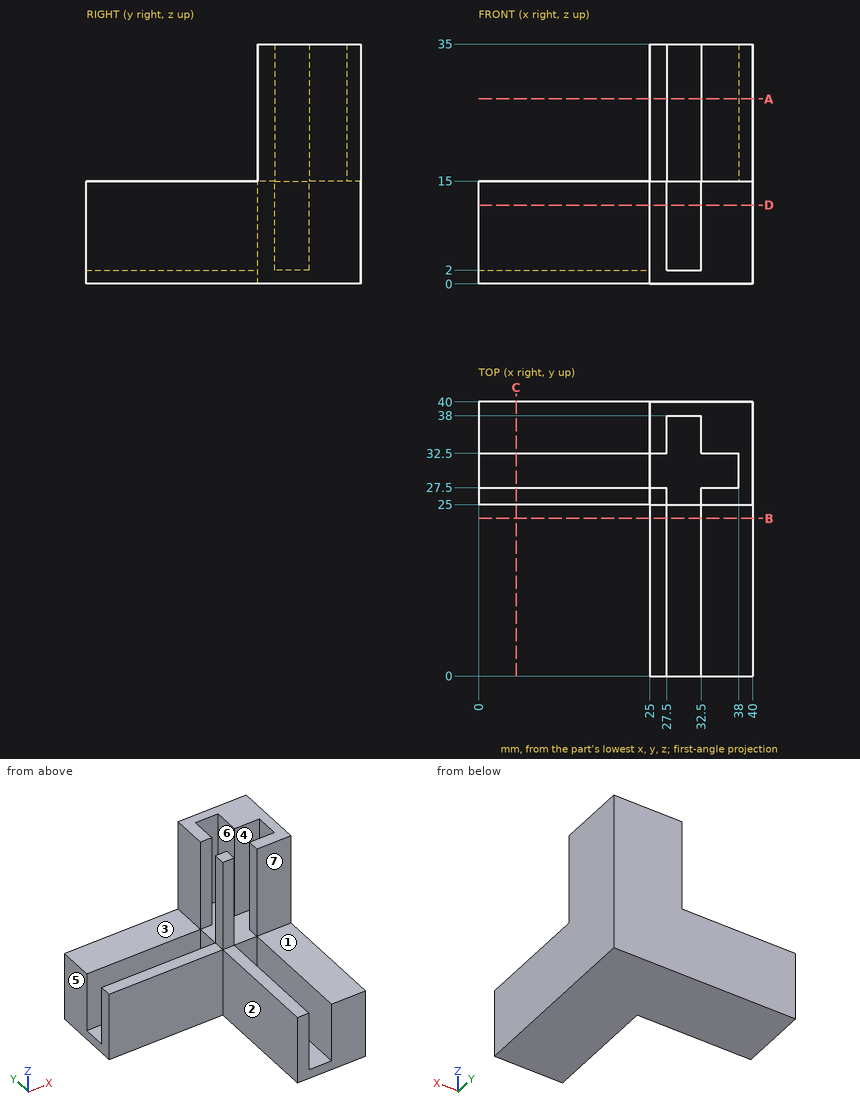
Answer from the drawing. Dimensions are ordinates in mm from the lowest x, y and z of the part. A direction names the side the tool comes from. Round coordinates to 2 decimals unless told otherwise and drop trailing zeros. Write each loop counter-clockwise with the first axis right and the second up, starting at its lowest first coordinate (ties: lowest second). Pieces come first, ordered by that corner, then holes. Notation, with made-up numbers: (-27, 52) -> (-6, 52) arc R17 ccw to (-6, 69) -> close; hole circle Ø6 at (74.25, 26). An arc over 180 degrees is marked (long way). Write each question's results on one line, items separated by ' | '.
1) The part is cut by section D-D (z = 11.5). Write down the section's boundary in (x, y), and give its area (3 significant figures).
Findings:
outline: (0, 25) -> (25, 25) -> (25, 0) -> (27.5, 0) -> (27.5, 25) -> (32.5, 25) -> (32.5, 0) -> (40, 0) -> (40, 40) -> (0, 40) -> (0, 32.5) -> (25, 32.5) -> (25, 27.5) -> (0, 27.5) -> close | area: 725 mm²
2) Which of the six approach directions +Z, -Z, +X, -X, +Y, -Y give full straight-line access (tool end or side, diameter ignored) to the marked faces 1, 2, 3 and 4?
Findings:
face 1: +Z, +X, -X, -Y | face 2: +Z, -Z, -X, -Y | face 3: +Z, -X, +Y, -Y | face 4: +Z, -X
3) The part is cut by section A-A (z = 27). Write down the section's boundary in (x, y).
Findings:
outline: (25, 25) -> (27.5, 25) -> (27.5, 27.5) -> (25, 27.5) -> close; (25, 32.5) -> (27.5, 32.5) -> (27.5, 38) -> (32.5, 38) -> (32.5, 32.5) -> (38, 32.5) -> (38, 27.5) -> (32.5, 27.5) -> (32.5, 25) -> (40, 25) -> (40, 40) -> (25, 40) -> close
4) Consider line 1 along X through (y, z) = (18, 6.5); line 2 along Z through (x, y) = (37, 21.5). Determine where each line is inside the solid, lowest interval first. Write a range as [from, to].
Findings:
line 1: x = [25, 27.5], [32.5, 40] | line 2: z = [0, 15]
5) For a pull along X with two mould halves and no side action, classify the marked faces 5, 6 and 7 as +X half, -X half, draft (parallel to the pull), parting line (faces both ways), or undercut.
Findings:
face 5: -X half | face 6: undercut | face 7: draft
6) The part is cut by section B-B (y = 23). Write down the section's boundary in (x, z), and give its area (3 significant figures).
Findings:
outline: (25, 0) -> (40, 0) -> (40, 15) -> (32.5, 15) -> (32.5, 2) -> (27.5, 2) -> (27.5, 15) -> (25, 15) -> close | area: 160 mm²
7) Flat-ended cylindrical pins translate along their axes: pin 1 (4.5 mm diameter, centred on y = 35.5, z = 24.5, fed in from -X); pin 2 (4 mm diameter, centred on x = 38, z = 27, fed in from -Y); pin 3 (1.5 mm diameter, centred on x = 7.5, y = 31, fed in from +Z). Find the tip coordinate at first contact, or state that the pin passes through.
Findings:
pin 1: stops at x = 25 | pin 2: stops at y = 25 | pin 3: stops at z = 2
